Input: dimensioned drawing with shaded views. Units: mm. Origin: part minimum x, y, z. Round coordinates to 2 decimals unless told otherwise and drop trailing zeros. Order: outer loops, then holes, each group sorted by start corner. A loop starts at its lowest first (then second) coordinate and runs counter-clockwise, first axis right, second up. Notation, with made-up numbers: (11, 50) - (25, 50) arc R20 cw to (25, 80) - close; hole circle Ø4 at (-32, 49). An arc over 180 degrees is marked (long way). Return JSON: item names as keys, results as strings. Group by question number.
1) Ray query, line 1 (Y direction, x = 35, z = 1); line 2 (X direction, y = 39.25, z = 1.5); line 3 (X direction, y = 56, z = 2.4) (1 decimal). Return the intervals inside material, ascending. Write a range as from..to.
2) Section A-A, the plane y = 56. Return loops of the section in (x, z) (1 decimal).
3) Section B-B, the plane y = 39.25. Give the number of separate pieces and of enclosed holes in the cut face, plus the area to 3 significant figures.
4) Contact query for flat-ended pins moving along their axis: P1, Ø2.5, axis at x = 23.825, y = 74.675, coming from the -Z side; P2, Ø1, axis at y = 19, z = 1.5, coming from the +X side. Output: stop coordinate, or through.
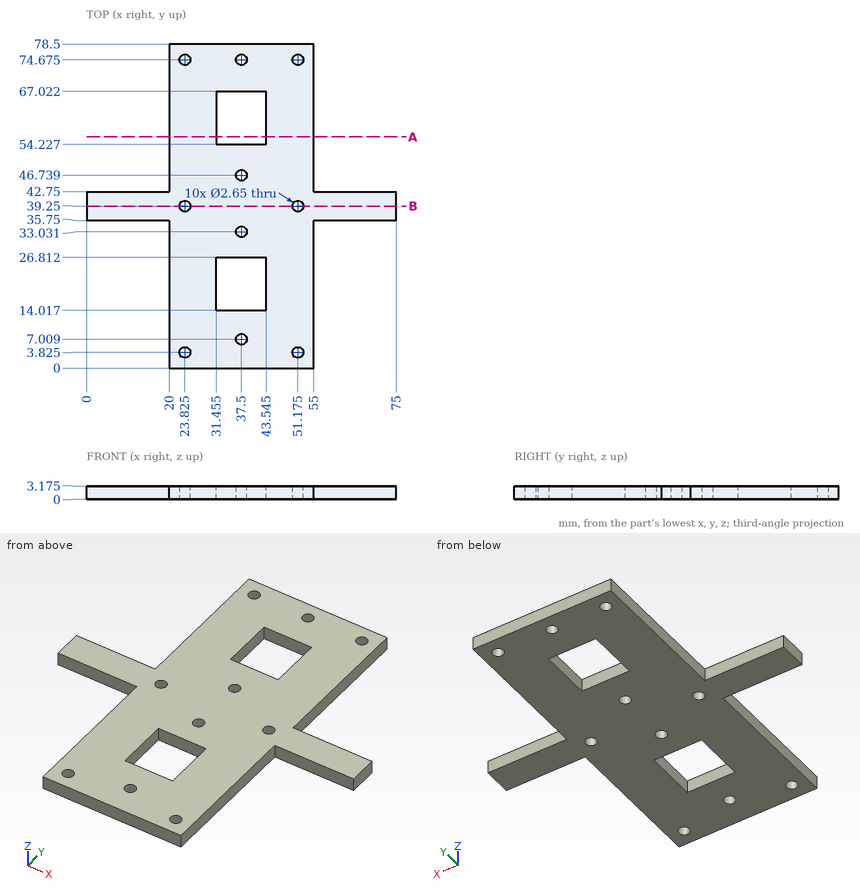
Geometry check:
{
 "1": {"line 1": "0..14.02, 26.81..54.23, 67.02..78.5", "line 2": "0..22.5, 25.15..49.85, 52.5..75", "line 3": "20..31.5, 43.5..55"},
 "2": {"outline": "(20, 0) - (31.5, 0) - (31.5, 3.2) - (20, 3.2) - close; (43.5, 0) - (55, 0) - (55, 3.2) - (43.5, 3.2) - close"},
 "3": {"separate pieces": "3", "enclosed holes": "0", "area": "221 mm2"},
 "4": {"P1": "through", "P2": "x = 55"}
}
